```python
from build123d import *

# Parameters (mm, degrees)
SKETCH1_R           = 24.1554
SKETCH1_R_2         = 20.32
BOSS_EXTRUDE1_DEPTH = 88.9
SKETCH2_R           = 4.7625
CUT_EXTRUDE1_DEPTH  = 33.5788
SKETCH3_R           = 4.7625
CUT_EXTRUDE2_DEPTH  = 33.5788


with BuildPart() as part:
    # Sketch1 → Boss-Extrude1 (new body)
    with BuildSketch(Plane(origin=(0, 0, 0), x_dir=(1, 0, 0), z_dir=(0, 1, 0))):
        Circle(SKETCH1_R)
        Circle(SKETCH1_R_2, mode=Mode.SUBTRACT)
    extrude(amount=BOSS_EXTRUDE1_DEPTH)

    # Sketch2 → Cut-Extrude1 (cut)
    with BuildSketch(Plane.XY):
        with Locations((0, 76.2)):
            Circle(SKETCH2_R)
    extrude(amount=-CUT_EXTRUDE1_DEPTH, mode=Mode.SUBTRACT)

    # Sketch3 → Cut-Extrude2 (cut)
    with BuildSketch(Plane(origin=(0, 0, 0), x_dir=(0, 0, -1), z_dir=(1, 0, 0))):
        with Locations((0, 69.85)):
            Circle(SKETCH3_R)
    extrude(amount=-CUT_EXTRUDE2_DEPTH, mode=Mode.SUBTRACT)


solid = part.part
```
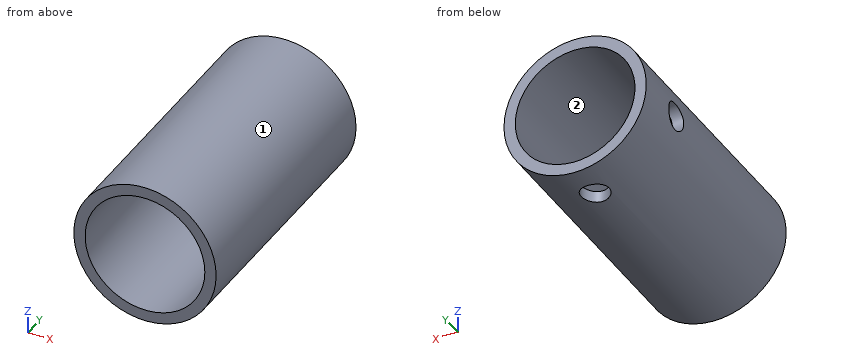
Check sheet for the modelled part. Datum: model origin and axes. Units: mm. Face numbers are marked on the shaded views. Give positions to 0.01 mm unless a question says otherwise; leave off trailing zeros. Order: outer loops, then holes, each group sorted by start corner. A loop starts at its lowest first (then second) coordinate and runs counter-clockwise, first axis right, second up. Notation, with made-up numbers: M -16.75,88 L 25.25,88 A22 ccw 25.25,115 Z; hole C 87.5,32.5 d5. An arc over 180 degrees is marked long. Answer in a Markdown table with one row per item.
1) Cross-section at B-B, the plane x = 0. Enter the section's corners in (y, z), plus the area to 3 significant figures.
Filled sheet:
| item | result |
|---|---|
| outline | M 0,-24.16 L 71.44,-24.16 L 71.44,-20.32 L 0,-20.32 Z; M 0,20.32 L 88.9,20.32 L 88.9,24.16 L 0,24.16 Z; M 80.96,-24.16 L 88.9,-24.16 L 88.9,-20.32 L 80.96,-20.32 Z |
| area | 645 mm2 |
2) Cross-section at A-A, the plane z = 0. Enter the section's corners in (x, y).
Filled sheet:
| item | result |
|---|---|
| outline | M -24.16,0 L -20.32,0 L -20.32,65.09 L -24.16,65.09 Z; M -24.16,74.61 L -20.32,74.61 L -20.32,88.9 L -24.16,88.9 Z; M 20.32,0 L 24.16,0 L 24.16,88.9 L 20.32,88.9 Z |
3) Release check for a two-part mould opening along X. For the marked faces 1 and 2 record: +X half, -X half, draft (parallel to the pull), parting line (faces both ways), or undercut.
Filled sheet:
| item | result |
|---|---|
| face 1 | parting line |
| face 2 | undercut |
4) Gauge pin test, flat ends, axial feed: P1, Ø10, axis at x = -16, y = 13.5, coming from the -Z side; P2, Ø4, axis at x = -11, y = 35, coming from the -Z side; P3, Ø15, axis at x = 0, y = 76.2, coming from the +Z side. Record the tip position at first contact, or that the pin passes through.
Filled sheet:
| item | result |
|---|---|
| P1 | stops at z = -21.51 |
| P2 | stops at z = -22.42 |
| P3 | stops at z = 24.16 |
5) Thickness scan on L1, parallel to X at y = 33, z = 0; L2, parallel to Y at x = 0, z = -23.2. Record the ranges inside material, lowest first. Write a range as [from, to].
Filled sheet:
| item | result |
|---|---|
| L1 | x = [-24.16, -20.32], [20.32, 24.16] |
| L2 | y = [0, 71.44], [80.96, 88.9] |
6) Cross-section at C-C, the plane x = 17.5. Enter the section's corners in (y, z), plus the area to 3 significant figures.
Filled sheet:
| item | result |
|---|---|
| outline | M 0,-16.65 L 88.9,-16.65 L 88.9,-10.33 L 0,-10.33 Z; M 0,10.33 L 88.9,10.33 L 88.9,16.65 L 0,16.65 Z |
| area | 1,120 mm2 |
7) Cross-section at D-D, the plane z = -17.5. Enter the section's corners in (x, y), plus the area to 3 significant figures.
Filled sheet:
| item | result |
|---|---|
| outline | M -16.65,0 L -10.33,0 L -10.33,88.9 L -16.65,88.9 Z; M 10.33,0 L 16.65,0 L 16.65,88.9 L 10.33,88.9 Z |
| area | 1,120 mm2 |
